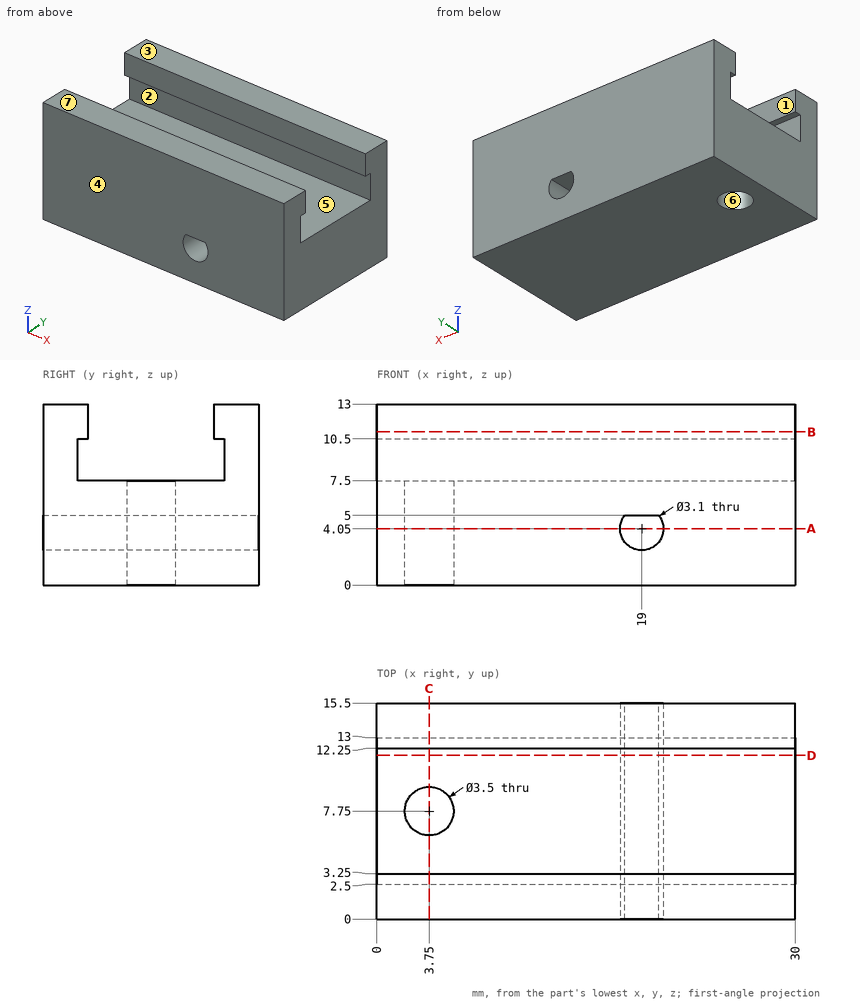
The figure shows three views and two pictorial views of one solid part (mm, origin at its lowest corner). Answer the questions. A direction names the side the tool comes from. Give positions to 0.01 mm unless a question says otherwise; leave off trailing zeros. Loops run counter-clockwise (first coordinate to the right, second up) from the corner with the lowest first, then second, coordinate; pieces in that order, holes last. Notation, with made-up numbers: (-27, -29.5) - (-17, -29.5) arc R26 ccw to (-17, 5.5) - close; hole circle Ø3 at (-39, 88.25). An arc over 180 degrees is marked (long way). Answer in a Markdown table with one row per item.
(1) A tool of negligible diameter and unlimited length cuts with its end or side. For the marked faces 1, 2 and 3, from which of +Z, -Z, +X, -X, +Y, -Y can it reach the whole face along a straight path? Write none if from no direction.
Results list:
| item | result |
|---|---|
| face 1 | +Z, +X, -X |
| face 2 | +X, -X |
| face 3 | +Z, +X, -X, +Y, -Y |
(2) Section A-A (z = 4.05) is taken. Give the vertices of the cut face in (x, y).
Results list:
| item | result |
|---|---|
| outline | (0, 0) - (17.45, 0) - (17.45, 15.5) - (0, 15.5) - close; (20.55, 0) - (30, 0) - (30, 15.5) - (20.55, 15.5) - close; hole circle Ø3.5 at (3.75, 7.75) |
(3) Consider L1, parallel to Z at x = 19, y = 6; L2, parallel to Y at x = 3.75, z = 5.5; L3, parallel to X at y = 14.75, z = 4. Determine where each line is inside the solid, lowest interval first. Write a range as [from, to].
Results list:
| item | result |
|---|---|
| L1 | z = [0, 2.5], [5, 7.5] |
| L2 | y = [0, 6], [9.5, 15.5] |
| L3 | x = [0, 17.45], [20.55, 30] |
(4) A flat-ended cylindrical pin translates along its axis: pin 1 Ø2 at (x, y) = (3.75, 7.75) entering from -Z. Find the tip coordinate at first contact, or state that the pin passes through.
Results list:
| item | result |
|---|---|
| pin 1 | passes through |
(5) Section B-B (z = 11) is taken. Give the vertices of the cut face in (x, y).
Results list:
| item | result |
|---|---|
| outline | (0, 0) - (30, 0) - (30, 3.25) - (0, 3.25) - close; (0, 12.25) - (30, 12.25) - (30, 15.5) - (0, 15.5) - close |
(6) Section C-C (x = 3.75) is taken. Give the vertices of the cut face in (y, z).
Results list:
| item | result |
|---|---|
| outline | (0, 0) - (6, 0) - (6, 7.5) - (2.5, 7.5) - (2.5, 10.5) - (3.25, 10.5) - (3.25, 13) - (0, 13) - close; (9.5, 0) - (15.5, 0) - (15.5, 13) - (12.25, 13) - (12.25, 10.5) - (13, 10.5) - (13, 7.5) - (9.5, 7.5) - close |
(7) For a pull along Y with two mould halves and no side action, classify the marked faces 4, 5, 6 and 7 as pulls with the +Y half, pulls with the -Y half, needs draft (parallel to the pull), parting line crosses it, or undercut.
Results list:
| item | result |
|---|---|
| face 4 | pulls with the -Y half |
| face 5 | undercut |
| face 6 | undercut |
| face 7 | needs draft |
(8) Section D-D (y = 11.75) is taken. Give the vertices of the cut face in (x, z).
Results list:
| item | result |
|---|---|
| outline | (0, 0) - (30, 0) - (30, 7.5) - (0, 7.5) - close; hole (17.78, 5) arc R1.55 ccw (long way) to (20.22, 5) - close |
